The listing builds one solid part. Answer for the finished solid, in the listing's coordinates (mm). A direction names the side the tool comes from. Give positions to 0.01 mm unless a question says otherwise; leave off trailing zeros. Order: outer loops, then holes, each group sorted by start corner. A loop starts at its lowest first (then second) coordinate and runs counter-clockwise, first axis right, second up.
```python
from build123d import *

# Parameters (mm, degrees)
F1_DEPTH = 2438.4


with BuildPart() as f1:
    # F0 (on Right) → F1 (new body)
    with BuildSketch(Plane.YZ):
        with BuildLine():
            Line((111.86897, 914.4), (0, 914.4))
            Line((0, 914.4), (0, 0))
            Line((0, 0), (1168.4, 0))
            Line((1168.4, 0), (1168.4, 289.752079))
            ThreePointArc((1168.4, 289.752079), (1146.081537, 343.633616), (1092.2, 365.952079))
            Line((1092.2, 365.952079), (508.629589, 365.952079))
            Line((508.629589, 365.952079), (289.065507, 1016))
            Line((289.065507, 1016), (111.86897, 1016))
            Line((111.86897, 1016), (111.86897, 914.4))
        make_face()
    extrude(amount=F1_DEPTH)


solid = f1.part
```
1) Find section A-A (x = 1034). Write down the section's boundary in (y, z).
Geometry says:
outline: (0, 0) - (1168.4, 0) - (1168.4, 289.75) arc R76.2 ccw to (1092.2, 365.95) - (508.63, 365.95) - (289.07, 1016) - (111.87, 1016) - (111.87, 914.4) - (0, 914.4) - close
2) Given P1, Ø6, axis at x = 1121.5, y = 750.5, coming from the +Z side, flat-ended and moving along its own axis, determine where the tip first touches the part or whether it passes through.
Geometry says:
P1: stops at z = 365.95
3) Find section B-B (y = 822.5). Write down the section's boundary in (x, z).
Geometry says:
outline: (0, 0) - (2438.4, 0) - (2438.4, 365.95) - (0, 365.95) - close
4) Straight lines are drawn through the part: probe 1 along Z at (x, y) = (530, 644); probe 2 along Y at (x, z) = (140.5, 390); probe 3 along Y at (x, z) = (1835.5, 793.5). For each, find the intervals that lie inside material, in ascending order.
Geometry says:
probe 1: z = 0 to 365.95
probe 2: y = 0 to 500.51
probe 3: y = 0 to 364.22
5) A tool of negligible diameter and unlimited length cuts with its end or side. For faces 1 (the flat face through (1202, 111.869, 966)), 2 (the flat face through (1202, 804, 365.952)), 3 (the flat face through (0, 446, 402)), from which of +Z, -Z, +X, -X, +Y, -Y can it reach the whole face along a straight path? Write none if from no direction.
Geometry says:
face 1: +Z, +X, -X, -Y
face 2: +Z, +X, -X, +Y
face 3: +Z, -Z, -X, +Y, -Y
6) Find section C-C (z = 644.5). Write down the section's boundary in (x, y).
Geometry says:
outline: (0, 0) - (2438.4, 0) - (2438.4, 414.55) - (0, 414.55) - close
